Autodesk Inventor part; units mm, degrees
ref_plane "pad_XY" through (0, 0, -12.7) normal (1, 0, 0) x (0, 0, -1)
ref_plane "pad_YZ" through (0, 0, -12.7) normal (0, 0, -1) x (0, 1, 0)
ref_plane "pad_ZX" through (0, 0, -12.7) normal (0, 1, 0) x (1, 0, 0)
sketch "Sketch_1" plane through (0, 0, 0) normal (0, 0, 1) x (1, 0, 0)
  line L0 (-6.35, 2.794) -> (-6.35, -2.794)
  arc A0 (-6.35, -2.794) -> (-5.969, -3.175) centre (-5.969, -2.794) ccw
  line L1 (-5.969, -3.175) -> (-4.191, -3.175)
  arc A1 (-3.81, -3.556) -> (-4.191, -3.175) centre (-4.191, -3.556) ccw
  line L2 (-3.81, -3.556) -> (-3.81, -9.9314)
  arc A2 (-3.81, -9.9314) -> (-3.429, -10.3124) centre (-3.429, -9.9314) ccw
  line L3 (-3.429, -10.3124) -> (-0.381, -10.3124)
  arc A3 (-0.381, -10.3124) -> (0, -9.9314) centre (-0.381, -9.9314) ccw
  line L4 (0, -9.9314) -> (0, 9.9314)
  arc A4 (0, 9.9314) -> (-0.381, 10.3124) centre (-0.381, 9.9314) ccw
  line L5 (-0.381, 10.3124) -> (-3.429, 10.3124)
  arc A5 (-3.429, 10.3124) -> (-3.81, 9.9314) centre (-3.429, 9.9314) ccw
  line L6 (-3.81, 9.9314) -> (-3.81, 3.556)
  arc A6 (-4.191, 3.175) -> (-3.81, 3.556) centre (-4.191, 3.556) ccw
  line L7 (-4.191, 3.175) -> (-5.969, 3.175)
  arc A7 (-5.969, 3.175) -> (-6.35, 2.794) centre (-5.969, 2.794) ccw
extrude "Extrusion1" add sketch "Sketch_1" along normal mid plane 47.371
sketch "Sketch_2" plane through (0, 0, 12.7) normal (0, 0, 1) x (1, 0, 0)
  line L0 (0, 0) -> (-6.35, 0)
  line L1 (-6.35, 0) -> (-6.35, 4.2164)
  line L2 (-6.35, 4.2164) -> (-4.1148, 4.2164)
  line L3 (-4.1148, 4.2164) -> (-2.463, 2.2479)
  line L4 (-2.463, 2.2479) -> (0, 2.2479)
  line L5 (0, 2.2479) -> (0, 0)
  line L6 (0, 0) -> (-6.35, 0)
revolve "Revolution1" cut sketch "Sketch_2" angle 360 about axis through (0, 0, 12.7) along (1, 0, 0)
sketch "Sketch_3" plane through (0, 0, -12.7) normal (0, 0, 1) x (1, 0, 0)
  line L0 (0, 0) -> (-6.35, 0)
  line L1 (-6.35, 0) -> (-6.35, 4.2164)
  line L2 (-6.35, 4.2164) -> (-4.1148, 4.2164)
  line L3 (-4.1148, 4.2164) -> (-2.463, 2.2479)
  line L4 (-2.463, 2.2479) -> (0, 2.2479)
  line L5 (0, 2.2479) -> (0, 0)
  line L6 (0, 0) -> (-6.35, 0)
revolve "Revolution2" cut sketch "Sketch_3" angle 360 about axis through (0, 0, -12.7) along (1, 0, 0)
sketch "Sketch_4" plane through (0, 0, 0) normal (1, 0, 0) x (0, 1, 0)
  line L0 (-3.175, 3.175) -> (-3.175, -3.175)
  line L1 (-3.175, -3.175) -> (3.175, -3.175)
  line L2 (3.175, -3.175) -> (3.175, 3.175)
  line L3 (3.175, 3.175) -> (-3.175, 3.175)
extrude "Extrusion2" cut sketch "Sketch_4" against normal blind 6.35
sketch "Sketch_5" plane through (0, 0, 0) normal (0, 0, 1) x (1, 0, 0)
  line L0 (-10.16, 6.35) -> (-10.16, -6.35)
  line L1 (-10.16, -6.35) -> (-3.81, -6.35)
  line L2 (-3.81, -6.35) -> (-3.81, 6.35)
  line L3 (-3.81, 6.35) -> (-10.16, 6.35)
extrude "Extrusion3" cut sketch "Sketch_5" along normal mid plane 6.35
ref_plane "pad_XY" through (0, 0, -12.7) normal (1, 0, 0) x (0, 0, -1)
ref_plane "pad_YZ" through (0, 0, -12.7) normal (0, 0, -1) x (0, 1, 0)
ref_plane "pad_ZX" through (0, 0, -12.7) normal (0, 1, 0) x (1, 0, 0)
ref_plane "s1_XY" through (-2.463, 0, 12.7) normal (1, 0, 0) x (0, 0, -1)
ref_plane "s1_YZ" through (-2.463, 0, 12.7) normal (0, 0, -1) x (0, 1, 0)
ref_plane "s1_ZX" through (-2.463, 0, 12.7) normal (0, 1, 0) x (1, 0, 0)
ref_plane "s2_XY" through (-2.463, 0, -12.7) normal (1, 0, 0) x (0, 0, -1)
ref_plane "s2_YZ" through (-2.463, 0, -12.7) normal (0, 0, -1) x (0, 1, 0)
ref_plane "s2_ZX" through (-2.463, 0, -12.7) normal (0, 1, 0) x (1, 0, 0)
properties part number "6705_p"
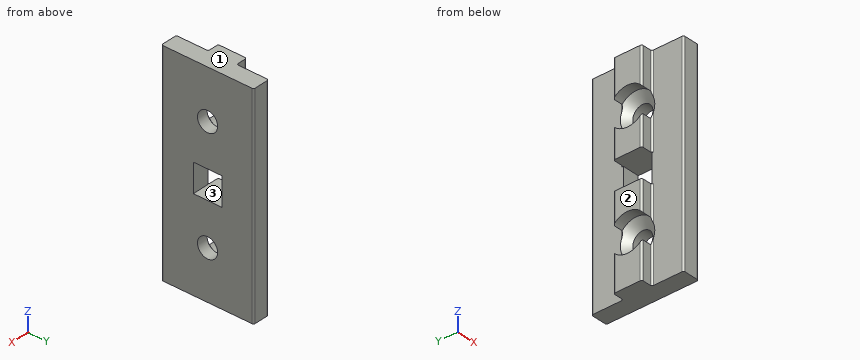
Design review of the part built by this model. Coordinates are the model's own, in mm. Face numbers are marked on the shaded views. Coordinates: 2 decimals unless noted, no trailing zeros. Order: outer loops, then holes, each group sorted by start corner. A loop starts at its lowest first (then second) coordinate and runs counter-clockwise, first axis right, second up.
1) Take a section at C-C, the plane y = 0. State how many separate pieces and enclosed holes the cut face has, and give its area (3 significant figures).
2) Take a section at A-A, the plane x = -4.75. Give the boundary of the cut face in (y, z) (1 decimal).
3) Mouldability with a two-part tool opening along Z and no side actions: class the marked faces 1, 2 and 3 as +Z half, -Z half, draft (parallel to the pull), parting line (faces both ways), or undercut.
4) Take a section at D-D, the plane z = -7. Give the boundary of the cut face in (x, y) (3 decimals), and give its area (3 significant figures).
5) Clearance check with flat-ended pins moving along their axes: pin 1 (0.9 mm diameter, centred on x = -5.5, z = -19.5, fed in from -Y) (3 decimals); pin 2 (0.5 mm diameter, centred on x = -5.5, z = 6.5, fed in from +Y) (3 decimals); pin 3 (1 mm diameter, centred on x = -3.5, z = -1.5, fed in from +Y); pin 4 (3 mm diameter, centred on y = -1, z = 13.5, fed in from -X). State where each tip first meets the part, or that it passes through.
6) Take a section at B-B, the plane z = 12.7. Give the boundary of the cut face in (x, y).
7) Wall thickness on line 1 along Z through (x, y) = (-0.8, 0) (1 decimal); line 2 along Z through (x, y) = (-2.5, -1.25) (1 decimal); line 3 along X through (y, z) = (3.75, -9): over which ranges is each line inside the solid? List them lowest first.
Returned:
1. separate pieces: 4
1. enclosed holes: 0
1. area: 179 mm2
2. outline: (-3.2, -23.7) - (3.2, -23.7) - (3.2, -15.5) arc R4.2 cw to (-3.2, -15.5) - close; (-3.2, -9.9) arc R4.2 cw to (3.2, -9.9) - (3.2, -3.2) - (-3.2, -3.2) - close; (-3.2, 3.2) - (3.2, 3.2) - (3.2, 9.9) arc R4.2 cw to (-3.2, 9.9) - close; (-3.2, 15.5) arc R4.2 cw to (3.2, 15.5) - (3.2, 23.7) - (-3.2, 23.7) - close
3. face 1: +Z half
3. face 2: draft
3. face 3: undercut
4. outline: (-6.35, -2.794) arc R0.381 ccw to (-5.969, -3.175) - (-4.191, -3.175) arc R0.381 cw to (-3.81, -3.556) - (-3.81, -9.931) arc R0.381 ccw to (-3.429, -10.312) - (-0.381, -10.312) arc R0.381 ccw to (0, -9.931) - (0, 9.931) arc R0.381 ccw to (-0.381, 10.312) - (-3.429, 10.312) arc R0.381 ccw to (-3.81, 9.931) - (-3.81, 3.556) arc R0.381 cw to (-4.191, 3.175) - (-5.969, 3.175) arc R0.381 ccw to (-6.35, 2.794) - close
4. area: 94.6 mm2
5. pin 1: stops at y = -3.175
5. pin 2: stops at y = 3.175
5. pin 3: stops at y = 10.31
5. pin 4: stops at x = -2.91
6. outline: (-3.81, -9.93) arc R0.38 ccw to (-3.43, -10.31) - (-0.38, -10.31) arc R0.38 ccw to (0, -9.93) - (0, -2.25) - (-2.46, -2.25) - (-3.81, -3.85) - close; (-3.81, 3.85) - (-2.46, 2.25) - (0, 2.25) - (0, 9.93) arc R0.38 ccw to (-0.38, 10.31) - (-3.43, 10.31) arc R0.38 ccw to (-3.81, 9.93) - close
7. line 1: z = -23.7 to -14.9, -10.5 to -3.2, 3.2 to 10.5, 14.9 to 23.7
7. line 2: z = -23.7 to -14.6, -10.8 to -3.2, 3.2 to 10.8, 14.6 to 23.7
7. line 3: x = -3.81 to 0
